from build123d import *

# Parameters (mm, degrees)
SKETCH1_R               = 7.5
SKETCH1_R_2             = 4.5
BOSS_EXTRUDE1_DEPTH     = 2
SKETCH1_2_R             = 4.5
BOSS_EXTRUDE2_DEPTH     = 55
CUT_EXTRUDE1_START      = -25
SKETCH2_R               = 4.5
CUT_EXTRUDE1_DEPTH      = 25
CUT_EXTRUDE2_DEPTH      = 25
CUT_EXTRUDE2_DEPTH_BACK = 25


with BuildPart() as part:
    # Sketch1 → Boss-Extrude1 (new body)
    with BuildSketch(Plane(origin=(0, 0, 0), x_dir=(1, 0, 0), z_dir=(0, 1, 0))):
        with Locations(Location((0, 0, 0), (0, 0, 270))):
            Circle(SKETCH1_R)
        with Locations(Location((0, 0, 0), (0, 0, 270))):
            Circle(SKETCH1_R_2, mode=Mode.SUBTRACT)
    extrude(amount=BOSS_EXTRUDE1_DEPTH)

    # Sketch1_2 → Boss-Extrude2 (add)
    with BuildSketch(Plane(origin=(0, 0, 0), x_dir=(1, 0, 0), z_dir=(0, 1, 0))):
        with Locations(Location((0, 0, 0), (0, 0, 270))):
            Circle(SKETCH1_2_R)
    extrude(amount=BOSS_EXTRUDE2_DEPTH)

    # Sketch2 → Cut-Extrude1 (cut)
    with BuildSketch(Plane(origin=(0, 55, 0), x_dir=(1, 0, 0), z_dir=(0, 1, 0)).offset(CUT_EXTRUDE1_START)):
        with Locations(Location((0, 0, 0), (0, 0, 270))):
            Circle(SKETCH2_R)
        with BuildLine():
            Line((-2, 1.811376185), (2, 1.811376185))
            ThreePointArc((2, 1.811376185), (2.698348325, 0), (2, -1.811376185))
            Line((2, -1.811376185), (-2, -1.811376185))
            ThreePointArc((-2, -1.811376185), (-2.698348325, 0), (-2, 1.811376185))
        make_face(mode=Mode.SUBTRACT)
    extrude(amount=CUT_EXTRUDE1_DEPTH, mode=Mode.SUBTRACT)

    # Sketch3 → Cut-Extrude2 (cut, two sides: drawn at the far end of the back side and taken through both)
    with BuildSketch(Plane(origin=(0, 0, -1.811376185), x_dir=(-1, 0, 0), z_dir=(0, 0, -1)).offset(-CUT_EXTRUDE2_DEPTH_BACK)):
        with BuildLine():
            ThreePointArc((1.75, 17.75), (1.237436867, 18.987436867), (0, 19.5))
            Line((0, 19.5), (0, 16))
            ThreePointArc((0, 16), (1.237436867, 16.512563133), (1.75, 17.75))
        make_face()
        with BuildLine():
            Line((0, 16), (0, 19.5))
            ThreePointArc((0, 19.5), (-1.75, 17.75), (0, 16))
        make_face()
        with BuildLine():
            ThreePointArc((1.75, 51.660798888), (1.237436867, 52.898235755), (0, 53.410798888))
            Line((0, 53.410798888), (0, 49.910798888))
            ThreePointArc((0, 49.910798888), (1.237436867, 50.423362021), (1.75, 51.660798888))
        make_face()
        with BuildLine():
            Line((0, 49.910798888), (0, 53.410798888))
            ThreePointArc((0, 53.410798888), (-1.75, 51.660798888), (0, 49.910798888))
        make_face()
    extrude(amount=CUT_EXTRUDE2_DEPTH + CUT_EXTRUDE2_DEPTH_BACK, mode=Mode.SUBTRACT)


solid = part.part
The listing builds one solid part. Answer for the finished solid, in the listing's coordinates (mm). A direction names the side the tool comes from. Round coordinates to 2 decimals unless told otherwise and drop trailing zeros. Order: outer loops, then holes, each group sorted by start corner. A loop starts at its lowest first (then second) coordinate and runs counter-clockwise, first axis right, second up. Notation, with made-up numbers: (-31.5, -22) - (12.5, -22) arc R19 cw to (12.5, -9) - close; hole circle Ø4 at (20.25, 36.25). An arc over 180 degrees is marked (long way). Write item = value, one per line. Start each with the question number.
1) Section D-D, the plane y = 45 is taken. Write down the section's boundary in (x, z), plus the area to 3 significant figures.
2) Straight lines are drawn through the part: L1, parallel to Y at x = 3.5, z = 3; L2, parallel to Z at x = 0.5, y = 35; L3, parallel to Y at x = -2.75, z = -2.5. For each, find the intervals that lie inside material, in ascending order.
3) Given pin 1 (4.5 mm diameter, centred on x = 0, y = 46.5, fed in from +Z); pin 2 (2 mm diameter, centred on y = 15.5, z = -3.5, fed in from -X); pin 3 (2 mm diameter, centred on x = -2.5, z = 4.5, fed in from +Y); pin 4 (1 mm diameter, centred on y = 37, z = -3, fed in from -X), each flat-ended and moving along its own axis, determine where each tip first touches the part or whether it passes through.
4) Section C-C, the plane z = 3.5 is taken. Write down the section's boundary in (x, y), plus the area to 3 significant figures.
5) For faces 1 (the cylindrical face through (2.7, 42.3, 0)), 2 (the flat face through (0, 30, 2)), 3 (the cylindrical face through (-2.7, 42.3, 0)), 4 (the flat face through (0, 42, -1.811)), 5 (the flat face through (0, 42, 1.811)), determine the directions among +Z, -Z, +X, -X, +Y, -Y from which every point of the face is accessible in a straight line to the end or side of a thin tool.
6) Section A-A, the plane z = 0 is taken. Write down the section's boundary in (x, y), plus the area to 3 significant figures.
7) Section B-B, the plane x = 1 is taken. Write down the section's boundary in (y, z).
Results list:
q1.outline = (-2, -1.81) - (2, -1.81) arc R2.7 ccw to (2, 1.81) - (-2, 1.81) arc R2.7 ccw to start
q1.area = 18.0 mm^2
q2.L1 = 0 to 2
q2.L2 = -1.81 to 1.81
q2.L3 = 0 to 30
q3.pin_1 = 1.81
q3.pin_2 = -3.74
q3.pin_3 = 30
q3.pin_4 = through
q4.outline = (-6.63, 0) - (6.63, 0) - (6.63, 2) - (2.83, 2) - (2.83, 30) - (-2.83, 30) - (-2.83, 2) - (-6.63, 2) - close; hole circle Ø3.5 at (0, 17.75)
q4.area = 175 mm^2
q5.face_1 = +X, +Y
q5.face_2 = +Y
q5.face_3 = -X, +Y
q5.face_4 = -Z, +X, -X, +Y
q5.face_5 = +Z, +X, -X, +Y
q6.outline = (-7.5, 0) - (7.5, 0) - (7.5, 2) - (4.5, 2) - (4.5, 30) - (2.7, 30) - (2.7, 55) - (-2.7, 55) - (-2.7, 30) - (-4.5, 30) - (-4.5, 2) - (-7.5, 2) - close; hole circle Ø3.5 at (0, 17.75); hole circle Ø3.5 at (0, 51.66)
q6.area = 398 mm^2
q7.outline = (0, -7.43) - (2, -7.43) - (2, -4.39) - (16.31, -4.39) - (16.31, 4.39) - (2, 4.39) - (2, 7.43) - (0, 7.43) - close; (19.19, -4.39) - (30, -4.39) - (30, -1.81) - (50.22, -1.81) - (50.22, 1.81) - (30, 1.81) - (30, 4.39) - (19.19, 4.39) - close; (53.1, -1.81) - (55, -1.81) - (55, 1.81) - (53.1, 1.81) - close
